For this review, take the finished solid that the model builds, in its own axes (mm). A direction names the side the tool comes from. Round coordinates to 2 decimals unless told otherwise and drop trailing zeros. Loops run counter-clockwise (first coordinate to the right, second up) from the corner with the lowest first, then second, coordinate; pieces in that order, holes last.
1. Consider section B-B on x = -1. State the section outline as (y, z) points, then the cut area to 3 significant figures.
2. Clearance check with flat-ended pins moving along their axes: pin 1 Ø4 at (y, z) = (-2.5, 7) entering from +X; pin 2 Ø0.5 at (y, z) = (-9.5, 7.5) entering from -X; pin 3 Ø1.2 at (y, z) = (-4.5, 9) entering from -X. State where each tip first meets the part, or that it passes through.
3. To check wall thickness, follow line 1 along Y through (x, z) = (0, 10.8) (3 decimals); line 2 along Y through (x, z) = (1.75, 5.25); line 3 along X through (y, z) = (-10, 5.25). State the ranges of each line that lie inside material, in increasing order.
4. Draft analysis for pull direction Z (two halves, no side actions). For faces 4 (the cylindrical face through (3.08, -7.6, 4.6)), 5 (the flat face through (2.8, -7, 9)), 6 (the flat face through (4, -7, 10.25)), 7 (the flat face through (-5.2, -7, 7)), state which applies: released by +Z, released by -Z, zero draft, split by the parting line, or undercut.
5. Consider section D-D on z = 8.5. State the section outline as (x, y) points (3 decimals), then the cut area to 3 significant figures.
6. Consider section A-A on y = -11. State the section outline as (x, z) points (3 decimals).
7. Tool access review of faces 1 (the flat face through (5.8, -7, 11)), 2 (the flat face through (-3, -11, 6)), 3 (the flat face through (-4, -7, 10.25)): name each direction out of +Z, -Z, +X, -X, +Y, -Y from which nothing blocks a thin tool from reaching the whole face with its end or side.
8. Consider section C-C on x = -3.25. State the section outline as (y, z) points.
from build123d import *

# Parameters (mm, degrees)
F1_DEPTH = 15
F2_R     = 3
F3_R     = 1.625
F4_DEPTH = 6
F6_DEPTH = 3


# Not quite as in the source:
# - a feature names something its author has since deleted; it is built from what else it names


with BuildPart() as f1:
    # F0 (on Front) → F1 (new body)
    with BuildSketch(Plane.XZ):
        Polygon((2.8, 7.8979998849), (2.8, 10), (2.8, 10.25), (5.8, 10.25), (5.8, 11.75), (0, 11.75), (-5.8, 11.75), (-5.8, 10.25), (-2.8, 10.25), (-2.8, 10), (-2.8, 7.8979998849), (-5.2, 7.8997776918), (-5.2, 6.8109772229), (-2.9620195233, 4.2), (0, 4.2), (2.9620195233, 4.2), (5.2, 6.8109772229), (5.2, 7.8997776918), align=None)
    extrude(amount=F1_DEPTH)

    # F2
    f2_edges = [f1.edges().sort_by_distance(p)[0] for p in [
        (-2.96202, -7.5, 4.2),
        (2.96202, -7.5, 4.2),
    ]]
    fillet(f2_edges, radius=F2_R)

    # F3 (on face) → F4 (cut)
    with BuildSketch(Plane.XY.offset(11.75)):
        with Locations((0, -4)):
            Circle(F3_R)
        with Locations((0, -11)):
            Circle(F3_R)
    extrude(amount=-F4_DEPTH, mode=Mode.SUBTRACT)

    # F5 (on face) → F6 (cut)
    with BuildSketch(Plane(origin=(0, 0, 4.2), x_dir=(1, 0, 0), z_dir=(0, 0, -1))):
        Polygon((3, 12.7320508076), (1.5822147558, 13.5506094999), (1.5822147558, 8.4493905001), (3, 9.2679491924), align=None)
        Polygon((-1.5822147558, 8.4493905001), (-1.5822147558, 13.5506094999), (-3, 12.7320508076), (-3, 9.2679491924), align=None)
        Polygon((-1.5822147558, 1.4493905001), (-1.5822147558, 6.5506094999), (-3, 5.7320508076), (-3, 2.2679491924), align=None)
        Polygon((3, 5.7320508076), (1.5822147558, 6.5506094999), (1.5822147558, 1.4493905001), (3, 2.2679491924), align=None)
        Polygon((1.5822147558, 13.5506094999), (0, 14.4641016151), (-1.5822147558, 13.5506094999), (-1.5822147558, 8.4493905001), (0, 7.5358983849), (1.5822147558, 8.4493905001), align=None)
        Polygon((1.5822147558, 1.4493905001), (1.5822147558, 6.5506094999), (0, 7.4641016151), (-1.5822147558, 6.5506094999), (-1.5822147558, 1.4493905001), (0, 0.5358983849), align=None)
    extrude(amount=-F6_DEPTH, mode=Mode.SUBTRACT)


solid = f1.part
Resolved:
1. outline: (-15, 4.2) - (-13.89, 4.2) - (-13.89, 7.2) - (-12.28, 7.2) - (-12.28, 11.75) - (-15, 11.75) - close; (-9.72, 7.2) - (-8.11, 7.2) - (-8.11, 4.2) - (-6.89, 4.2) - (-6.89, 7.2) - (-5.28, 7.2) - (-5.28, 11.75) - (-9.72, 11.75) - close; (-2.72, 7.2) - (-1.11, 7.2) - (-1.11, 4.2) - (0, 4.2) - (0, 11.75) - (-2.72, 11.75) - close
1. area: 55.3 mm2
2. pin 1: stops at x = 5.2
2. pin 2: stops at x = -5.2
2. pin 3: stops at x = -2.8
3. line 1: y = -15 to -12.625, -9.375 to -5.625, -2.375 to 0
3. line 2: y = -15 to -13.45, -8.55 to -6.45, -1.55 to 0
3. line 3: x = -3.86 to -3, 3 to 3.86
4. face 4: released by -Z
4. face 5: undercut
4. face 6: undercut
4. face 7: zero draft
5. outline: (-2.8, -15) - (2.8, -15) - (2.8, 0) - (-2.8, 0) - close; hole circle Ø3.25 at (0, -11); hole circle Ø3.25 at (0, -4)
5. area: 67.4 mm2
6. outline: (-5.8, 10.25) - (-2.8, 10.25) - (-2.8, 7.898) - (-5.2, 7.9) - (-5.2, 6.811) - (-3.86, 5.248) arc R3 ccw to (-3, 4.556) - (-3, 7.2) - (-1.625, 7.2) - (-1.625, 11.75) - (-5.8, 11.75) - close; (1.625, 7.2) - (3, 7.2) - (3, 4.556) arc R3 ccw to (3.86, 5.248) - (5.2, 6.811) - (5.2, 7.9) - (2.8, 7.898) - (2.8, 10.25) - (5.8, 10.25) - (5.8, 11.75) - (1.625, 11.75) - close
7. face 1: +Z, -Z, +X, +Y, -Y
7. face 2: -Z
7. face 3: -X, +Y, -Y
8. outline: (-15, 4.71) - (0, 4.71) - (0, 7.9) - (-15, 7.9) - close; (-15, 10.25) - (0, 10.25) - (0, 11.75) - (-15, 11.75) - close
